The drawing under review shows one solid part. Ordinate dimensions are in mm from its lowest x, y, z. A direction names the side the tool comes from. Coordinates: 2 decimals unless noted, no trailing zeros. Write each loop counter-clockwise with the first axis right and the second up, starting at its lowest first coordinate (ties: lowest second). Pieces come first, ordered by that corner, then holes. Notation, with made-up numbers: (-23, -12.5) -> (7, -12.5) arc R23 ccw to (7, 22.5) -> close; hole circle Ø11 at (-17.5, -34.75). An arc over 180 degrees is marked (long way). Put each result on its own line as item: value. Start each with the question number.
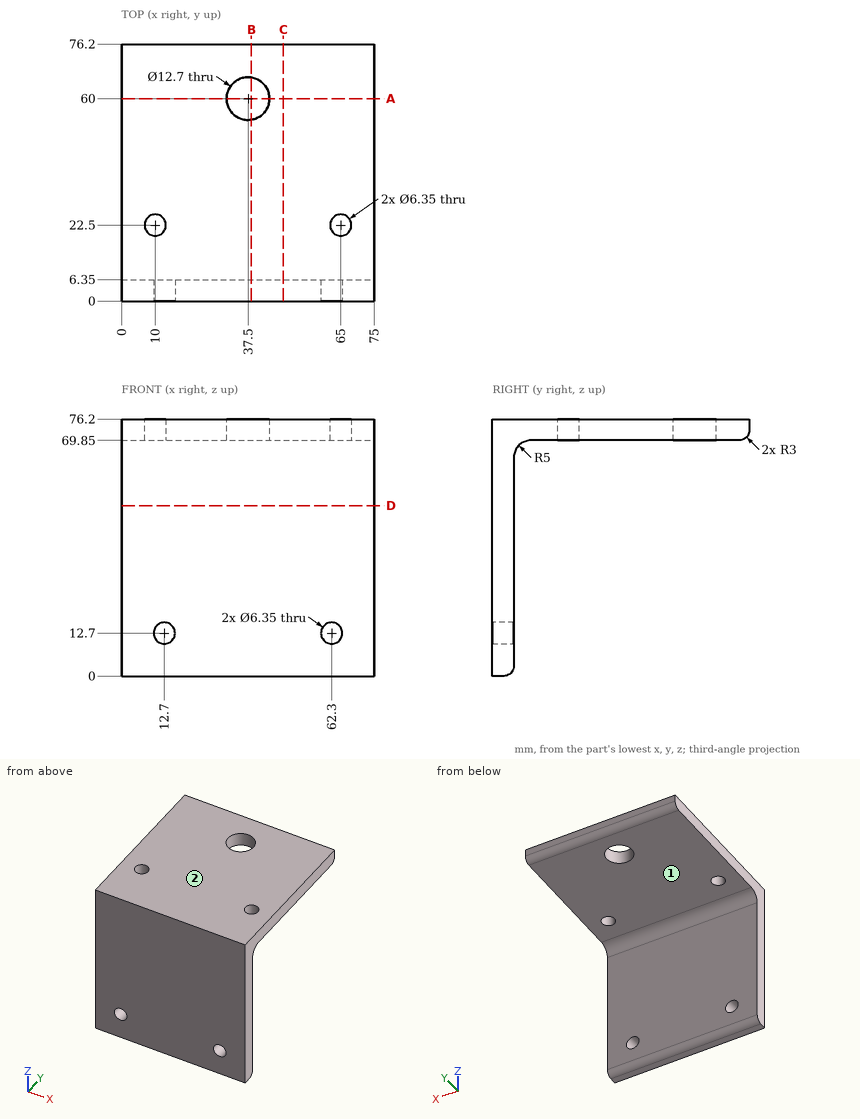
1. Consider section C-C on x = 48. State the section outline as (y, z) points, then the cut area to 3 significant figures.
2. Consider section A-A on y = 60. State the section outline as (x, z) points, then the cut area to 3 significant figures.
3. Consider section B-B on x = 38.5. State the section outline as (y, z) points, then the cut area to 3 significant figures.
4. Consider section D-D on z = 50.5. State the section outline as (x, y) points, then the cut area to 3 significant figures.
5. Wall thickness on line 1 (X direction, y = 2.5, z = 12.7) (3 decimals); line 2 (Y direction, x = 65, z = 74.75) (3 decimals); line 3 (Y direction, x = 37.5, z = 74.75): over which ranges is each line inside the solid? List them lowest first. Write a range as from..to.
6. Insertion check: P1, Ø8.5, axis at x = 10, y = 22.5, coming from the -Z side; P2, Ø8.5, axis at x = 62.3, z = 12.7, coming from the +Y side; P3, Ø5, axis at x = 18.5, z = 35.5, coming from the -Y side; P4, Ø7.5, axis at x = 37.5, y = 60, coming from the -Z side. Each pin has a flat end and moves straight along its axis. Give the tip position at first contact, or say it passes through.
7. Tool access review of the marked faces 1 and 2: name each direction out of +Z, -Z, +X, -X, +Y, -Y from which nothing blocks a thin tool from reaching the whole face with its end or side.
Output values:
1. outline: (0, 0) -> (3.35, 0) arc R3 ccw to (6.35, 3) -> (6.35, 64.85) arc R5 cw to (11.35, 69.85) -> (73.2, 69.85) arc R3 ccw to (76.2, 72.85) -> (76.2, 76.2) -> (0, 76.2) -> close
1. area: 929 mm^2
2. outline: (0, 69.85) -> (31.15, 69.85) -> (31.15, 76.2) -> (0, 76.2) -> close; (43.85, 69.85) -> (75, 69.85) -> (75, 76.2) -> (43.85, 76.2) -> close
2. area: 396 mm^2
3. outline: (0, 0) -> (3.35, 0) arc R3 ccw to (6.35, 3) -> (6.35, 64.85) arc R5 cw to (11.35, 69.85) -> (53.73, 69.85) -> (53.73, 76.2) -> (0, 76.2) -> close; (66.27, 69.85) -> (73.2, 69.85) arc R3 ccw to (76.2, 72.85) -> (76.2, 76.2) -> (66.27, 76.2) -> close
3. area: 849 mm^2
4. outline: (0, 0) -> (75, 0) -> (75, 6.35) -> (0, 6.35) -> close
4. area: 476 mm^2
5. line 1: x = 0..9.525, 15.875..59.125, 65.475..75
5. line 2: y = 0..19.325, 25.675..76.2
5. line 3: y = 0..53.65, 66.35..76.2
6. P1: stops at z = 69.85
6. P2: stops at y = 6.35
6. P3: stops at y = 0
6. P4: passes through
7. face 1: -Z, +X, -X, +Y
7. face 2: +Z, +X, -X, +Y, -Y
